```python
from build123d import *

# Parameters (mm, degrees)
SKETCH_W     = 34
SKETCH_H     = 89
PAD_DEPTH    = 10
PAD001_DEPTH = 7
PAD002_DEPTH = 7


with BuildPart() as part:
    # Sketch → Pad (new body)
    with BuildSketch(Plane.XY):
        Polygon((-22, 0), (-18, 0), (-18, -5), (18, -5), (18, 0), (22, 0), (22, 4.25), (21.5, 4.25), (21.5, 5.25), (24, 5.25), (24, -100), (-24, -100), (-24, 5.25), (-21.5, 5.25), (-21.5, 4.25), (-22, 4.25), align=None)
        with Locations((0, -53.5)):
            Rectangle(SKETCH_W, SKETCH_H, mode=Mode.SUBTRACT)
    extrude(amount=PAD_DEPTH)

    # Sketch001 (on DatumPlane) → Pad001 (join)
    with BuildSketch(Plane.YZ.offset(-17)):
        with BuildLine():
            Line((-100, 0), (-100, 30))
            Line((-95, 30), (-100, 30))
            ThreePointArc((-95, 30), (-88.049566, 10.375362), (-70, 0))
            Line((-100, 0), (-70, 0))
        make_face()
    extrude(amount=-PAD001_DEPTH)

    # Sketch002 (on DatumPlane) → Pad002 (join)
    with BuildSketch(Plane.YZ.offset(17)):
        with BuildLine():
            Line((-100, 0), (-100, 30))
            Line((-95, 30), (-100, 30))
            ThreePointArc((-95, 30), (-88.049566, 10.375362), (-70, 0))
            Line((-100, 0), (-70, 0))
        make_face()
    extrude(amount=PAD002_DEPTH)


solid = part.part
```
The model under review builds one solid part; all positions refer to its coordinate system, in mm. A direction names the side the tool comes from. Round coordinates to 2 decimals unless told otherwise and drop trailing zeros. Order: outer loops, then holes, each group sorted by start corner. A loop starts at its lowest first (then second) coordinate and runs counter-clockwise, first axis right, second up.
Item 1: Draft analysis for pull direction Y (two halves, no side actions). For faces 6 (the flat face through (24, -47, 5)), 7 (the flat face through (22, 2, 5)), 8 (the flat face through (0, -98, 5)), 9 (the flat face through (0, -5, 5)), state which applies: released by +Y, released by -Y, zero draft, split by the parting line, or undercut.
Working result:
face 6: zero draft
face 7: undercut
face 8: undercut
face 9: released by +Y
Item 2: Add section D-D, the plane y = -7.5. State the section outline as (x, z) points, and give its area (3 significant figures).
Working result:
outline: (-24, 0) - (24, 0) - (24, 10) - (-24, 10) - close
area: 480 mm2
Item 3: Add section C-C, the plane z = 7.5. State the section outline as (x, y) points.
Working result:
outline: (-24, -100) - (24, -100) - (24, 5.25) - (21.5, 5.25) - (21.5, 4.25) - (22, 4.25) - (22, 0) - (18, 0) - (18, -5) - (-18, -5) - (-18, 0) - (-22, 0) - (-22, 4.25) - (-21.5, 4.25) - (-21.5, 5.25) - (-24, 5.25) - close; hole (-17, -98) - (17, -98) - (17, -9) - (-17, -9) - close
Item 4: Machinability: for faces 1 (the flat face through (0, -99, 10)), 2 (the flat face through (18, -3, 5)), 3 (the flat face through (18, -38, 10)), 4 (the flat face through (-24, -60, 8)), 5 (the flat face through (-22, 2, 5)), which of the approach directions +Z, -Z, +X, -X, +Y, -Y give a long, thin tool a straight path to every point of the face, cutting with its end or side? Answer none if there is none.
Working result:
face 1: +Z, +Y, -Y
face 2: +Z, -Z, +Y
face 3: +Z, +X, -X, +Y
face 4: +Z, -Z, -X, +Y, -Y
face 5: +Z, -Z
Item 5: To check wall thickness, follow probe 1 along X at (y, z) = (-37, 4.25); probe 2 along Y at (x, z) = (4, 5.5); probe 3 along Y at (x, z) = (-19, 11.5). State the ranges of each line that lie inside material, in increasing order.
Working result:
probe 1: x = -24 to -17, 17 to 24
probe 2: y = -100 to -98, -9 to -5
probe 3: y = -100 to -88.94
Item 6: For pin 1 (1.2 mm diameter, centred on x = 19.5, z = 2.5, fed in from +Y); pin 2 (1.5 mm diameter, centred on x = 19, y = -74.5, fed in from +Z); pin 3 (8 mm diameter, centred on x = 3, z = 3.5, fed in from +Y); pin 4 (10 mm diameter, centred on y = -64, z = 17, fed in from +X), all flat-tipped, find the tip position at first contact; note any pin that passes through.
Working result:
pin 1: stops at y = 0
pin 2: stops at z = 10
pin 3: stops at y = -5
pin 4: passes through
Item 7: Add section A-A, the plane y = -31. State the section outline as (x, z) points.
Working result:
outline: (-24, 0) - (-17, 0) - (-17, 10) - (-24, 10) - close; (17, 0) - (24, 0) - (24, 10) - (17, 10) - close
Item 8: Add section B-B, the plane x = -2. State the section outline as (y, z) points, and give its area (3 significant figures).
Working result:
outline: (-100, 0) - (-98, 0) - (-98, 10) - (-100, 10) - close; (-9, 0) - (-5, 0) - (-5, 10) - (-9, 10) - close
area: 60.0 mm2
